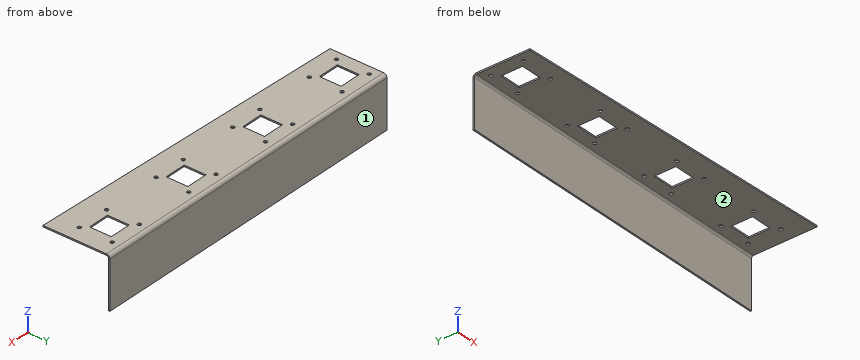
Autodesk Inventor part; units mm, degrees
ref_plane "YZ Plane" through (0, 0, 0) normal (1, 0, 0) x (0, 1, 0)
ref_plane "XZ Plane" through (0, 0, 0) normal (0, 1, 0) x (-1, 0, 0)
ref_plane "XY Plane" through (0, 0, 0) normal (0, 0, 1) x (1, 0, 0)
sketch "Sketch1" plane through (0, 0, 0) normal (0, 0, 1) x (1, 0, 0)
  line L0 (0, 0) -> (-470, 0)
  line L1 (0, -94) -> (0, 0)
  line L2 (-470, 0) -> (-470, -80)
  line L3 (-470, -80) -> (0, -94)
  point P0 (0, -47)
  dimension "d32" = 94
  dimension "d60" = 80
  dimension "d61" = 470
extrude "Plate1" add sketch "Sketch1" along normal blind 2
sketch "Sketch8" plane through (0, 0, 2) normal (0, 0, 1) x (1, 0, 0)
  line L0 (-29.75, -53.25) -> (-60.25, -53.25)
  line L1 (-60.25, -53.25) -> (-60.25, -22.75)
  line L2 (-60.25, -22.75) -> (-29.75, -22.75)
  line L3 (-29.75, -22.75) -> (-29.75, -53.25)
  line L4 (-29.75, -53.25) -> (-60.25, -22.75) construction
  line L5 (-60.25, -53.25) -> (-29.75, -22.75) construction
  circle A0 centre (-22, -61) radius 2.5
  circle A1 centre (-68, -61) radius 2.5
  circle A2 centre (-68, -15) radius 2.5
  circle A3 centre (-22, -15) radius 2.5
  line L6 (0, 0) -> (0, -94)
  line L7 (-470, 0) -> (0, 0)
  line L8 (-60.25, -53.25) -> (-68, -61) construction
  line L9 (-68, -15) -> (-22, -15) construction
  line L10 (-22, -15) -> (-22, -61) construction
  line L11 (-22, -61) -> (-68, -61) construction
  line L12 (-68, -61) -> (-68, -15) construction
  point P0 (-45, -38)
  dimension "d51" = 30.5
  dimension "d52" = 30.5
  dimension "d53" = 5
  dimension "d72" = 45
  dimension "d78" = 46
  dimension "d79" = 15
extrude "Cut3" cut sketch "Sketch8" against normal blind 2
pattern_linear "Rectangular Pattern1" count 4 spacing 130 along (-1, 0, 0) of "Cut3"
sketch "Sketch9" plane through (0, -2, 2) normal (0, 1, 0) x (-1, 0, 0)
  line L0 (470, 0) -> (0, 0)
  line L1 (0, 0) -> (0, -72)
  line L2 (0, -72) -> (470, -72)
  line L3 (470, -72) -> (470, 0)
edge flange "Flange3" height 72 angle 90 thickness 2 bend radius 2.75 thickness toward (0, 1, 0) relief round relief width 2 relief depth 1 edges at (-235, 0, 0) wall of the first edge with corners at (-470, -2, 2) (0, -2, 2) (0, -2, -70) (-470, -2, -70)
bend "Bend3"
corner "Corner3"
equation "\"d51\" = d52"
equation "\"d55\" = Thickness"
equation "\"d2\" = Thickness"
equation "\"d62\" = BendReliefWidth"
equation "\"d63\" = BendReliefDepth"
equation "\"d64\" = MinimumRemnant"
equation "\"d65\" = TransitionRadius"
equation "\"d68\" = BendRadius"
equation "\"d69\" = CornerReliefSize"
equation "\"d70\" = GapSize"
equation "\"d71\" = JacobiRadiusSize"
equation "\"BendReliefWidth\" = Thickness"
equation "\"BendReliefDepth\" = 0.5 * Thickness"
equation "\"CornerReliefSize\" = 4 * Thickness"
equation "\"MinimumRemnant\" = 2 * Thickness"
equation "\"TransitionRadius\" = BendRadius"
equation "\"JacobiRadiusSize\" = BendRadius"
equation "\"GapSize\" = Thickness"
properties part number "PRS 1422 DrSysB diameter way up_1200" material "Stainless Steel"
Build history of the part. All positions in model axes, mm. Face numbers are marked on the shaded views. A direction names the side the tool comes from. Round coordinates to 2 decimals unless told otherwise and drop trailing zeros. Order: outer loops, then holes, each group sorted by start corner. A loop starts at its lowest first (then second) coordinate and runs counter-clockwise, first axis right, second up. Notation, with made-up numbers: (-4, -10.75) -> (0, -10.75) arc R29 cw to (0, 26.25) -> close; hole circle Ø11 at (42.25, 40). An arc over 180 degrees is marked (long way). Answer in a Markdown table with one row per item.
1) Which spindle directions (+Z, -Z, +X, -X, +Y, -Y) get a long thin tool onto all of the face, cutting with end or side? Do the marked faces 1 and 2. Say none if no direction does.
Values:
| item | result |
|---|---|
| face 1 | +Z, -Z, +X, -X, +Y |
| face 2 | -Z, +X, -X, -Y |
2) Band-saw the part on B-B on z = -22. Give the cut face in (x, y).
Values:
| item | result |
|---|---|
| outline | (-470, -2) -> (0, -2) -> (0, 0) -> (-470, 0) -> close |
3) Pin check, flat tips, straight feed: P1, Ø1, axis at x = -264.5, z = -55, coming from the -Y side; P2, Ø10, axis at x = -216, y = -28.5, coming from the -Z side; P3, Ø2, axis at x = -302.5, z = 1, coming from the +Y side. Stop position of each tip, or through.
Values:
| item | result |
|---|---|
| P1 | y = -2 |
| P2 | z = 0 |
| P3 | y = -0.88 |
4) Band-saw the part on D-D on y = -73.5. Give the cut face in (x, z).
Values:
| item | result |
|---|---|
| outline | (-470, 0) -> (0, 0) -> (0, 2) -> (-470, 2) -> close |
5) Wall check: L1, parallel to Y at x = -282, z = 0.95; L2, parallel to Y at x = -458, z = 1.3; L3, parallel to Z at x = -306, y = -65.5. Give the ranges that are in metal, low to high.
Values:
| item | result |
|---|---|
| L1 | -85.6 to -63.5, -58.5 to -17.5, -12.5 to -1.77 |
| L2 | -80.36 to -63.5, -58.5 to -17.5, -12.5 to -2.27 |
| L3 | 0 to 2 |
6) Band-saw the part on C-C on x = -387. Give the cut face in (y, z), and give its area (3 significant figures).
Values:
| item | result |
|---|---|
| outline | (-82.47, 0) -> (-4.75, 0) arc R2.75 cw to (-2, -2.75) -> (-2, -70) -> (0, -70) -> (0, -2.75) arc R4.75 ccw to (-4.75, 2) -> (-82.47, 2) -> close |
| area | 302 mm2 |
7) Band-saw the part on A-A on x = -302.5. Give the cut face in (y, z).
Values:
| item | result |
|---|---|
| outline | (-84.99, 0) -> (-53.25, 0) -> (-53.25, 2) -> (-84.99, 2) -> close; (-22.75, 0) -> (-4.75, 0) arc R2.75 cw to (-2, -2.75) -> (-2, -70) -> (0, -70) -> (0, -2.75) arc R4.75 ccw to (-4.75, 2) -> (-22.75, 2) -> close |
